Autodesk Inventor part; units mm, degrees
ref_plane "YZ Plane" through (0, 0, 0) normal (1, 0, 0) x (0, 1, 0)
ref_plane "XZ Plane" through (0, 0, 0) normal (0, 1, 0) x (-1, 0, 0)
ref_plane "XY Plane" through (0, 0, 0) normal (0, 0, 1) x (1, 0, 0)
sketch "Sketch1" plane through (0, 0, 0) normal (0, 1, 0) x (-1, 0, 0)
  circle A0 centre (56.9406, -14.9623) radius 2.3241
  circle A1 centre (66.6693, -6.7989) radius 2.3241
  circle A2 centre (41.2693, -6.7989) radius 2.3241
  circle A3 centre (-41.6882, -6.7989) radius 2.3241
  circle A4 centre (-57.3594, -14.9623) radius 2.3241
  circle A5 centre (-67.0882, -6.7989) radius 2.3241
  arc A6 (-59.7156, -7.3708) -> (-58.0844, -7.6169) centre (-58.6976, -6.1526) ccw
  line L0 (-59.7156, -7.3708) -> (-85.288, 13.999)
  arc A7 (-43.7185, -2.4382) -> (-58.0844, -7.6169) centre (0.2546, -146.9346) ccw
  arc A8 (-43.7185, -2.4382) -> (-37.2086, 0.6056) centre (-51.1134, 21.8615) ccw
  arc A9 (-69.7478, -12.8722) -> (-69.4607, -10.2448) centre (-70.4786, -11.4629) ccw
  line L1 (-99.204, 14.6104) -> (-69.4607, -10.2448)
  arc A10 (-69.7478, -12.8722) -> (-78.2828, -17.6558) centre (-0.2094, -146.9516) ccw
  arc A11 (-16.3345, 6.2393) -> (-15.3068, 3.3313) centre (-15.4655, 4.9108) ccw
  arc A12 (14.8879, 3.3313) -> (-15.3068, 3.3313) centre (-0.2094, -146.9516) ccw
  arc A13 (14.8879, 3.3313) -> (15.9157, 6.2393) centre (15.0466, 4.9108) ccw
  arc A14 (37.2538, 0.5886) -> (43.7637, -2.4551) centre (51.1586, 21.8446) ccw
  arc A15 (58.1296, -7.6339) -> (43.7637, -2.4551) centre (-0.2094, -146.9516) ccw
  line L2 (85.3331, 13.982) -> (59.7607, -7.3877)
  arc A16 (58.1296, -7.6339) -> (59.7607, -7.3877) centre (58.7428, -6.1696) ccw
  line L3 (69.0418, -10.2448) -> (98.7851, 14.6104)
  arc A17 (69.0418, -10.2448) -> (69.3289, -12.8722) centre (70.0598, -11.4629) ccw
  arc A18 (77.8639, -17.6558) -> (69.3289, -12.8722) centre (-0.2094, -146.9516) ccw
  line L4 (66.6693, -6.7989) -> (41.2693, -6.7989)
  line L5 (0, 0) -> (0, 4.0875)
  circle A19 centre (66.6693, -6.7989) radius 3.9782
  circle A20 centre (41.2693, -6.7989) radius 4.9026
  line L6 (66.6693, -2.8207) -> (41.4483, -1.8996)
  circle A21 centre (56.9406, -14.9623) radius 4.1852
  line L7 (69.4813, -9.613) -> (60.0669, -17.7447)
  line L8 (54.6165, -18.4429) -> (39.1949, -11.241)
  line L9 (56.9406, -14.9623) -> (56.9406, -141.9623)
  arc A22 (56.9406, -141.9623) -> (36.3667, -6.7989) centre (-501.2889, -157.7854) ccw
  line L10 (56.9406, -141.9623) -> (75.9906, -141.9623)
  line L11 (75.9906, -141.9623) -> (75.9906, -17.7447)
  line L12 (75.9906, -17.7447) -> (65.708, -12.8722)
  circle A23 centre (-66.6693, -6.7989) radius 3.9782
  circle A24 centre (-41.2693, -6.7989) radius 4.9026
  line L13 (-66.6693, -2.8207) -> (-41.4483, -1.8996)
  circle A25 centre (-56.9406, -14.9623) radius 4.1852
  line L14 (-69.4813, -9.613) -> (-60.0669, -17.7447)
  arc A26 (-36.3667, -6.7989) -> (-56.9406, -141.9623) centre (501.2889, -157.7854) ccw
  line L15 (-56.9406, -141.9623) -> (-75.9906, -141.9623)
  line L16 (-75.9906, -141.9623) -> (-75.9906, -17.7447)
  line L17 (-75.9906, -17.7447) -> (-65.708, -12.8722)
  arc A27 (42.2115, -1.9275) -> (-42.2115, -1.9275) centre (0, -148.5156) ccw
  arc A28 (39.6774, -11.4417) -> (-39.7321, -11.4576) centre (0, -148.5156) ccw
  point P0 (-37.4811, -10.825)
  point P1 (37.4811, -10.825)
  dimension "d0" = 127
  dimension "d1" = 19.05
extrude "Extrusion1" add sketch "Sketch1" along normal blind 1.5875 contours L0 L13 A8 A7 A6 | A6 A7 A8 A24 A26 L15 L16 L17 L14 A23 L13 L0 | A23 L14 | L13 A24 A8 | A27 L6 A20 A22 A28 A26 A24 L13 | A24 A26 | A26 A24 | L6 L2 L4 A15 A14 | A14 A20 L6 | A14 A15 L4 A20 | A20 A22 | L6 A19 L2 | A28 L8 A21 L9 A22 | A22 A20 L8 A28 | L4 A15 A16 L2 A19 L7 A21 L8 A20 | A22 A20 | A19 L4 L2 | A19 L7 | L9 A21 L7 L12 L11 L10 | L4 L2 A16 A15 | A21 | A25 picked at (-63.4219, -7.1214) picked at (63.3048, -7.3068)
fillet "Fillet1" radius 38.1 2 edges at (37.4811, 0.7937, -10.825) (-37.4811, 0.7937, -10.825)
sketch "Sketch2" plane through (0, 1.5875, 0) normal (0, 1, 0) x (1, 0, 0)
  line L0 (0, 0) -> (0, -4.0291)
  arc A0 (-42.2115, 1.9275) -> (42.2115, 1.9275) centre (0, 148.5156) ccw
  line L1 (42.2115, 1.9275) -> (66.6693, 2.8207)
  arc A1 (66.6693, 2.8207) -> (69.4813, 9.613) centre (66.6693, 6.7989) ccw
  line L2 (69.4813, 9.613) -> (65.708, 12.8722)
  line L3 (65.708, 12.8722) -> (75.9906, 17.7447)
  line L4 (75.9906, 17.7447) -> (75.9906, 141.9623)
  line L5 (75.9906, 141.9623) -> (56.9406, 141.9623)
  arc A2 (43.6777, 35.794) -> (56.9406, 141.9623) centre (-501.2889, 157.7854) ccw
  arc A3 (8.8646, 6.0903) -> (43.6777, 35.794) centre (6.4979, 44.1168) ccw
  arc A4 (-8.8646, 6.0903) -> (8.8646, 6.0903) centre (0, 148.5156) ccw
  arc A5 (-43.6777, 35.794) -> (-8.8646, 6.0903) centre (-6.4979, 44.1168) ccw
  arc A6 (-56.9406, 141.9623) -> (-43.6777, 35.794) centre (501.2889, 157.7854) ccw
  line L6 (-56.9406, 141.9623) -> (-75.9906, 141.9623)
  line L7 (-75.9906, 141.9623) -> (-75.9906, 17.7447)
  line L8 (-75.9906, 17.7447) -> (-65.708, 12.8722)
  line L9 (-65.708, 12.8722) -> (-69.4813, 9.613)
  arc A7 (-69.4813, 9.613) -> (-66.6693, 2.8207) centre (-66.6693, 6.7989) ccw
  line L10 (-66.6693, 2.8207) -> (-42.2115, 1.9275)
  arc A8 (-42.2115, 1.9275) -> (42.2115, 1.9275) centre (0, 148.5156) ccw
  circle A9 centre (-41.2693, 6.7989) radius 2.3241
  circle A10 centre (-66.6693, 6.7989) radius 2.3241
  circle A11 centre (57.3594, 14.9623) radius 2.3241
  circle A12 centre (67.0882, 6.7989) radius 2.3241
  circle A13 centre (41.6882, 6.7989) radius 2.3241
  circle A14 centre (-56.9406, 14.9623) radius 2.3241
  circle A15 centre (67.0882, 6.7989) radius 6.35
  line L11 (73.2907, 5.4382) -> (75.9906, 17.7447)
  line L12 (42.2115, 1.9275) -> (66.7086, 0.4603)
  circle A16 centre (-67.0882, 6.7989) radius 6.35
  line L13 (-73.2907, 5.4382) -> (-75.9906, 17.7447)
  line L14 (-42.2115, 1.9275) -> (-66.7086, 0.4603)
  point P0 (-42.2115, 1.9275)
  dimension "d5" = 12.7
extrude "Extrusion2" add sketch "Sketch2" against normal blind 1.5875 contours L14 A16 L10 | A16 L8 L9 A7 L10 | L1 A15 L12 | L13 L8 A16 | L1 A1 L2 L3 A15 | L3 L11 A15 picked at (-67.6214, 11.869) picked at (67.6293, 11.8682)
sketch "Sketch3" plane through (0, 1.5875, 0) normal (0, 1, 0) x (1, 0, 0)
  line L0 (75.9906, 17.7447) -> (75.9906, 141.9623)
  line L1 (75.9906, 141.9623) -> (56.9406, 141.9623)
  arc A0 (43.6777, 35.794) -> (56.9406, 141.9623) centre (-501.2889, 157.7854) ccw
  arc A1 (8.8646, 6.0903) -> (43.6777, 35.794) centre (6.4979, 44.1168) ccw
  arc A2 (-8.8646, 6.0903) -> (8.8646, 6.0903) centre (0, 148.5156) ccw
  arc A3 (-43.6777, 35.794) -> (-8.8646, 6.0903) centre (-6.4979, 44.1168) ccw
  arc A4 (-56.9406, 141.9623) -> (-43.6777, 35.794) centre (501.2889, 157.7854) ccw
  line L2 (-56.9406, 141.9623) -> (-75.9906, 141.9623)
  line L3 (-75.9906, 141.9623) -> (-75.9906, 17.7447)
  line L4 (-75.9906, 17.7447) -> (-73.2907, 5.4382)
  arc A5 (-73.2907, 5.4382) -> (-66.7086, 0.4603) centre (-67.0882, 6.7989) ccw
  line L5 (-66.7086, 0.4603) -> (-42.2115, 1.9275)
  arc A6 (-42.2115, 1.9275) -> (42.2115, 1.9275) centre (0, 148.5156) ccw
  line L6 (42.2115, 1.9275) -> (66.7086, 0.4603)
  arc A7 (66.7086, 0.4603) -> (73.2907, 5.4382) centre (67.0882, 6.7989) ccw
  line L7 (73.2907, 5.4382) -> (75.9906, 17.7447)
  circle A8 centre (-41.2693, 6.7989) radius 2.3241
  circle A9 centre (-66.6693, 6.7989) radius 2.3241
  circle A10 centre (57.3594, 14.9623) radius 2.3241
  circle A11 centre (67.0882, 6.7989) radius 2.3241
  circle A12 centre (41.6882, 6.7989) radius 2.3241
  circle A13 centre (-56.9406, 14.9623) radius 2.3241
  line L8 (-75.9906, 141.9623) -> (-75.9906, 17.7447)
  line L9 (75.9906, 17.7447) -> (-75.9906, 17.7447)
  line L10 (-75.9906, 17.7447) -> (0, 17.7447)
  line L11 (0, 17.7447) -> (0, 5.8147)
  arc A14 (-8.8646, 6.0903) -> (8.8646, 6.0903) centre (0, 148.5156) ccw
  line L12 (8.8646, 141.9623) -> (-8.8646, 141.9623)
  line L13 (8.8646, 141.9623) -> (15.2146, 141.9623)
  line L14 (-8.8646, 141.9623) -> (-15.2146, 141.9623)
  line L15 (-15.2146, 141.9623) -> (-15.2146, 7.0273)
  line L16 (15.2146, 141.9623) -> (15.2146, 7.0273)
  point P0 (0, 0)
  dimension "d8" = 6.35
  dimension "d9" = 6.35
extrude "Extrusion3" add sketch "Sketch3" against normal blind 1.5875 contours A1 A2 L11 L9 L16 | L9 L15 L14 L12 L13 L16 | L11 A2 A3 L15 L9
sketch "Sketch4" plane through (0, 1.5875, 0) normal (0, 1, 0) x (1, 0, 0)
  line L0 (75.9906, 17.7447) -> (75.9906, 141.9623)
  line L1 (75.9906, 141.9623) -> (56.9406, 141.9623)
  arc A0 (43.6777, 35.794) -> (56.9406, 141.9623) centre (-501.2889, 157.7854) ccw
  arc A1 (15.2146, 7.0273) -> (43.6777, 35.794) centre (6.4979, 44.1168) ccw
  line L2 (15.2146, 7.0273) -> (15.2146, 141.9623)
  line L3 (15.2146, 141.9623) -> (-15.2146, 141.9623)
  line L4 (-15.2146, 141.9623) -> (-15.2146, 7.0273)
  arc A2 (-43.6777, 35.794) -> (-15.2146, 7.0273) centre (-6.4979, 44.1168) ccw
  arc A3 (-56.9406, 141.9623) -> (-43.6777, 35.794) centre (501.2889, 157.7854) ccw
  line L5 (-56.9406, 141.9623) -> (-75.9906, 141.9623)
  line L6 (-75.9906, 141.9623) -> (-75.9906, 17.7447)
  line L7 (-75.9906, 17.7447) -> (-73.2907, 5.4382)
  arc A4 (-73.2907, 5.4382) -> (-66.7086, 0.4603) centre (-67.0882, 6.7989) ccw
  line L8 (-66.7086, 0.4603) -> (-42.2115, 1.9275)
  arc A5 (-42.2115, 1.9275) -> (42.2115, 1.9275) centre (0, 148.5156) ccw
  line L9 (42.2115, 1.9275) -> (66.7086, 0.4603)
  arc A6 (66.7086, 0.4603) -> (73.2907, 5.4382) centre (67.0882, 6.7989) ccw
  line L10 (73.2907, 5.4382) -> (75.9906, 17.7447)
  circle A7 centre (-41.2693, 6.7989) radius 2.3241
  circle A8 centre (-66.6693, 6.7989) radius 2.3241
  circle A9 centre (57.3594, 14.9623) radius 2.3241
  circle A10 centre (67.0882, 6.7989) radius 2.3241
  circle A11 centre (41.6882, 6.7989) radius 2.3241
  circle A12 centre (-56.9406, 14.9623) radius 2.3241
  line L11 (-15.2146, 44.1168) -> (15.2146, 44.1168)
  line L12 (15.2146, 44.1168) -> (15.2146, 75.8668)
  line L13 (15.2146, 75.8668) -> (52.8576, 88.5598)
  arc A13 (43.6777, 35.794) -> (56.9406, 141.9623) centre (-501.2889, 157.7854) ccw
  line L14 (15.2146, 75.8668) -> (15.2146, 94.9168)
  line L15 (15.2146, 141.9623) -> (15.2146, 7.0273)
  line L16 (15.2146, 94.9168) -> (54.9699, 108.3221)
  line L17 (0, 44.1168) -> (0, 50.0619)
  line L18 (-15.2146, 75.8668) -> (-52.8576, 88.5598)
  line L19 (-15.2146, 94.9168) -> (-54.9699, 108.3221)
  point P0 (0, 0)
  dimension "d12" = 31.75
  dimension "d13" = 19.05
extrude "Extrusion4" add sketch "Sketch4" against normal blind 1.5875 contours A0 L13 L2 L16 | L4 L18 A3 L19
sketch "Sketch5" plane through (0, 1.5875, 0) normal (0, 1, 0) x (1, 0, 0)
  arc A0 (43.6777, 35.794) -> (52.8576, 88.5598) centre (-501.2889, 157.7854) ccw
  arc A1 (15.2146, 7.0273) -> (43.6777, 35.794) centre (6.4979, 44.1168) ccw
  line L0 (15.2146, 7.0273) -> (15.2146, 75.8668)
  line L1 (15.2146, 75.8668) -> (52.8576, 88.5598)
  line L2 (54.9699, 108.3221) -> (15.2146, 94.9168)
  line L3 (15.2146, 94.9168) -> (15.2146, 141.9623)
  line L4 (15.2146, 141.9623) -> (-15.2146, 141.9623)
  line L5 (-15.2146, 141.9623) -> (-15.2146, 94.9168)
  line L6 (-15.2146, 94.9168) -> (-54.9699, 108.3221)
  arc A2 (-56.9406, 141.9623) -> (-54.9699, 108.3221) centre (501.2889, 157.7854) ccw
  line L7 (-56.9406, 141.9623) -> (-75.9906, 141.9623)
  line L8 (-75.9906, 141.9623) -> (-75.9906, 17.7447)
  line L9 (-75.9906, 17.7447) -> (-73.2907, 5.4382)
  arc A3 (-73.2907, 5.4382) -> (-66.7086, 0.4603) centre (-67.0882, 6.7989) ccw
  line L10 (-66.7086, 0.4603) -> (-42.2115, 1.9275)
  arc A4 (-42.2115, 1.9275) -> (42.2115, 1.9275) centre (0, 148.5156) ccw
  line L11 (42.2115, 1.9275) -> (66.7086, 0.4603)
  arc A5 (66.7086, 0.4603) -> (73.2907, 5.4382) centre (67.0882, 6.7989) ccw
  line L12 (73.2907, 5.4382) -> (75.9906, 17.7447)
  line L13 (75.9906, 17.7447) -> (75.9906, 141.9623)
  line L14 (75.9906, 141.9623) -> (56.9406, 141.9623)
  arc A6 (54.9699, 108.3221) -> (56.9406, 141.9623) centre (-501.2889, 157.7854) ccw
  line L15 (-52.8576, 88.5598) -> (-15.2146, 75.8668)
  line L16 (-15.2146, 75.8668) -> (-15.2146, 7.0273)
  arc A7 (-43.6777, 35.794) -> (-15.2146, 7.0273) centre (-6.4979, 44.1168) ccw
  arc A8 (-52.8576, 88.5598) -> (-43.6777, 35.794) centre (501.2889, 157.7854) ccw
  circle A9 centre (-41.2693, 6.7989) radius 2.3241
  circle A10 centre (-66.6693, 6.7989) radius 2.3241
  circle A11 centre (57.3594, 14.9623) radius 2.3241
  circle A12 centre (67.0882, 6.7989) radius 2.3241
  circle A13 centre (41.6882, 6.7989) radius 2.3241
  circle A14 centre (-56.9406, 14.9623) radius 2.3241
  line L17 (-42.2115, 1.9275) -> (-42.2115, -17.1225)
  line L18 (-70.5723, 1.4901) -> (-42.2115, -17.1225)
  line L19 (0, 0) -> (0, -4.0291)
  arc A15 (-73.2907, 5.4382) -> (-66.7086, 0.4603) centre (-67.0882, 6.7989) ccw
  line L20 (42.2115, 1.9275) -> (42.2115, -17.1225)
  line L21 (70.5723, 1.4901) -> (42.2115, -17.1225)
  line L22 (-42.2115, -17.1225) -> (42.2115, -17.1225)
  dimension "d16" = 19.05
extrude "Extrusion5" add sketch "Sketch5" against normal blind 1.5875 contours L21 L20 L11 A5 | L22 L17 A4 L20 | L18 A3 L10 L17
properties part number "ABS Intake Hood"
Verification items for the finished model (mm, model axes). A direction names the side the tool comes from. Coordinates: 2 decimals unless noted, no trailing zeros. Loops run counter-clockwise (first coordinate to the right, second up) from the corner with the lowest first, then second, coordinate; pieces in that order, holes last. Notation, with made-up numbers: (31, 83.25) -> (62, 83.25) arc R21 ccw to (62, 97.25) -> close; hole circle Ø4 at (46.5, -6.5). An arc over 180 degrees is marked (long way). Put each result on its own line as item: value.
1. Section check C-C, the plane y = 0.8. Give the number of separate pieces and of enclosed holes in the cut face, then the cut area to 3 significant figures.
Result set:
separate pieces: 1
enclosed holes: 8
area: 15,800 mm^2
2. Mould release check, pull along Z, two halves, no side actions. Record for faces 1 (the face through (56.59, 0.805, 7.686)), 2 (the face through (34.814, 0.805, -101.526)), 3 (the face through (64.871, 0.783, -7.497)): pulls with the +Z half, pulls with the -Z half, needs draft (parallel to the pull), parting line crosses it, or undercut.
Result set:
face 1: pulls with the +Z half
face 2: pulls with the -Z half
face 3: undercut
3. Section check B-B, the plane z = -43. Record the boundary of the cut face in (x, y), then the cut area to 3 significant figures.
Result set:
outline: (-75.99, 0) -> (-45.24, 0) -> (-45.24, 1.59) -> (-75.99, 1.59) -> close; (-15.21, 0) -> (15.21, 0) -> (15.21, 1.59) -> (-15.21, 1.59) -> close; (45.24, 0) -> (75.99, 0) -> (75.99, 1.59) -> (45.24, 1.59) -> close
area: 146 mm^2
4. Section check D-D, the plane z = 2. Record the boundary of the cut face in (x, y), then the cut area to 3 significant figures.
Result set:
outline: (-65.25, 0) -> (65.25, 0) -> (65.25, 1.59) -> (-65.25, 1.59) -> close
area: 207 mm^2
5. Thickness scan on line 1 (X direction, y = 0.7, z = -33); line 2 (X direction, y = 0.7, z = -54); line 3 (Z direction, x = 21, y = 0.55). Record the ranges inside material, lowest first.
Result set:
line 1: x = -75.99 to -42.94, -15.21 to 15.21, 42.94 to 75.99
line 2: x = -75.99 to -47.44, -15.21 to 15.21, 47.44 to 75.99
line 3: z = -96.87 to -77.82, -8.88 to 17.12
6. Tool access check on faces 4 (the face through (1, 0, -61)), 5 (the face through (-33.773, 0.805, -82.124)), 6 (the face through (-34.814, 0.805, -101.526)). Record the directions out of +Z, -Z, +X, -X, +Y, -Y that give a thin tool (end or side, any length) a straight path to the whole face; none if there is none.
Result set:
face 4: +Z, -Z, +X, -X, -Y
face 5: +Y, -Y
face 6: -Z, +Y, -Y
7. Section check A-A, the plane z = -130. Record the boundary of the cut face in (x, y), then the cut area to 3 significant figures.
Result set:
outline: (-75.99, 0) -> (-56.47, 0) -> (-56.47, 1.59) -> (-75.99, 1.59) -> close; (-15.21, 0) -> (15.21, 0) -> (15.21, 1.59) -> (-15.21, 1.59) -> close; (56.47, 0) -> (75.99, 0) -> (75.99, 1.59) -> (56.47, 1.59) -> close
area: 110 mm^2
